Geometry check sheet. Reference: the model listing, model coordinates, mm. Round coordinates to 2 decimals unless told otherwise and drop trailing zeros. Loops run counter-clockwise (first coordinate to the right, second up) from the corner with the lowest first, then second, coordinate; pieces in that order, holes last. Notation, with made-up numbers: M 49,-24.5 L 105,-24.5 A8 cw 105,-11.5 Z; hole C -28.5,-13.5 d11. An arc over 180 degrees is marked long. Use one line per item in the form item = value. Start each with the question number.
1. Cross-section at C-C (z = 0.3). Record the boundary of the cut face in (x, y).
2. Material ranges on line 1 (Y direction, x = -37, z = 0.6); line 2 (X direction, y = 64.5, z = 0.35); line 3 (Y direction, x = -14.5, z = 1.35), recorded low to high.
3. Cross-section at B-B (y = 68.5). Record the boundary of the cut face in (x, z), then the cut area to 3 significant figures.
4. Cross-section at A-A (x = -23.5). Record the boundary of the cut face in (y, z).
5. Go/stop test with a flat-tipped pin: pin 1 (10 mm diameter, centred on x = -35, y = 28.5, fed in from -Z). Record where the tip stops, or that it passes through.
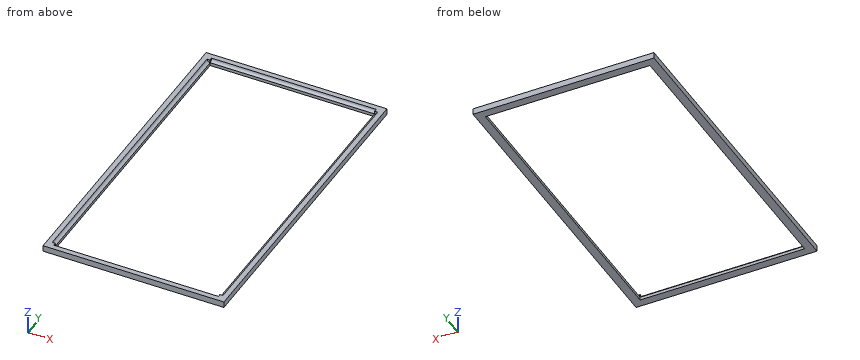
```python
from build123d import *

# Parameters (mm, degrees)
F1_DEPTH = 1.5
F4_DEPTH = 40.341
F5_DEPTH = 74


with BuildPart() as f1:
    # F0 (on Top) → F1 (new body)
    with BuildSketch(Plane.XY):
        Polygon((-44.341, 78), (-44.341, 15.8245135099), (-42.341, 15.8245135099), (-42.341, 76), (-24.9481573701, 76), (-24.9481573701, 78), align=None)
        Polygon((-44.341, 0), (0, 0), (0, 78), (-24.9481573701, 78), (-24.9481573701, 76), (-2, 76), (-2, 2), (-42.341, 2), (-42.341, 15.8245135099), (-44.341, 15.8245135099), align=None)
    extrude(amount=F1_DEPTH)

    # F2 (on face) → F4 (cut)
    with BuildSketch(Plane.YZ.offset(-42.341)):
        with BuildLine():
            ThreePointArc((76, 0.75), (76.5303300859, 0.9696699141), (76.75, 1.5))
            ThreePointArc((76.75, 1.5), (76, 2.25), (75.25, 1.5))
            Line((75.25, 1.5), (76, 1.5))
            Line((76, 1.5), (76, 0.75))
        make_face()
        with BuildLine():
            Line((76, 1.5), (75.25, 1.5))
            ThreePointArc((75.25, 1.5), (75.4696699141, 0.9696699141), (76, 0.75))
            Line((76, 0.75), (76, 1.5))
        make_face()
        with BuildLine():
            Line((2, 1.5), (2.75, 1.5))
            ThreePointArc((2.75, 1.5), (1.4696699141, 2.0303300859), (2, 0.75))
            Line((2, 0.75), (2, 1.5))
        make_face()
        with BuildLine():
            ThreePointArc((2, 0.75), (2.5303300859, 0.9696699141), (2.75, 1.5))
            Line((2.75, 1.5), (2, 1.5))
            Line((2, 1.5), (2, 0.75))
        make_face()
    extrude(amount=F4_DEPTH, mode=Mode.SUBTRACT)

    # F3 (on face) → F5 (cut)
    with BuildSketch(Plane.XZ.offset(-76)):
        with BuildLine():
            Line((-42.341, 1.5), (-41.591, 1.5))
            ThreePointArc((-41.591, 1.5), (-42.8713300859, 2.0303300859), (-42.341, 0.75))
            Line((-42.341, 0.75), (-42.341, 1.5))
        make_face()
        with BuildLine():
            ThreePointArc((-42.341, 0.75), (-41.8106699141, 0.9696699141), (-41.591, 1.5))
            Line((-41.591, 1.5), (-42.341, 1.5))
            Line((-42.341, 1.5), (-42.341, 0.75))
        make_face()
        with BuildLine():
            ThreePointArc((-1.25, 1.5), (-2, 2.25), (-2.75, 1.5))
            Line((-2.75, 1.5), (-2, 1.5))
            Line((-2, 1.5), (-2, 0.75))
            ThreePointArc((-2, 0.75), (-1.4696699141, 0.9696699141), (-1.25, 1.5))
        make_face()
        with BuildLine():
            Line((-2, 1.5), (-2.75, 1.5))
            ThreePointArc((-2.75, 1.5), (-2.5303300859, 0.9696699141), (-2, 0.75))
            Line((-2, 0.75), (-2, 1.5))
        make_face()
    extrude(amount=F5_DEPTH, mode=Mode.SUBTRACT)


solid = f1.part
```
Reported:
q1.outline = M -44.34,0 L 0,0 L 0,78 L -44.34,78 Z; hole M -42.34,2 L -2,2 L -2,76 L -42.34,76 Z
q2.line_1 = 0 to 2, 76 to 78
q2.line_2 = -44.34 to -42.34, -2 to 0
q2.line_3 = 0 to 1.27, 76.73 to 78
q3.outline = M -44.34,0 L -42.34,0 L -42.34,0.75 A0.75 cw -43.09,1.5 L -44.34,1.5 Z; M -2,0 L 0,0 L 0,1.5 L -1.25,1.5 A0.75 cw -2,0.75 Z
q3.area = 5.12 mm²
q4.outline = M 0,0 L 2,0 L 2,0.75 A0.75 cw 1.25,1.5 L 0,1.5 Z; M 76,0 L 78,0 L 78,1.5 L 76.75,1.5 A0.75 cw 76,0.75 Z
q5.pin_1 = through
